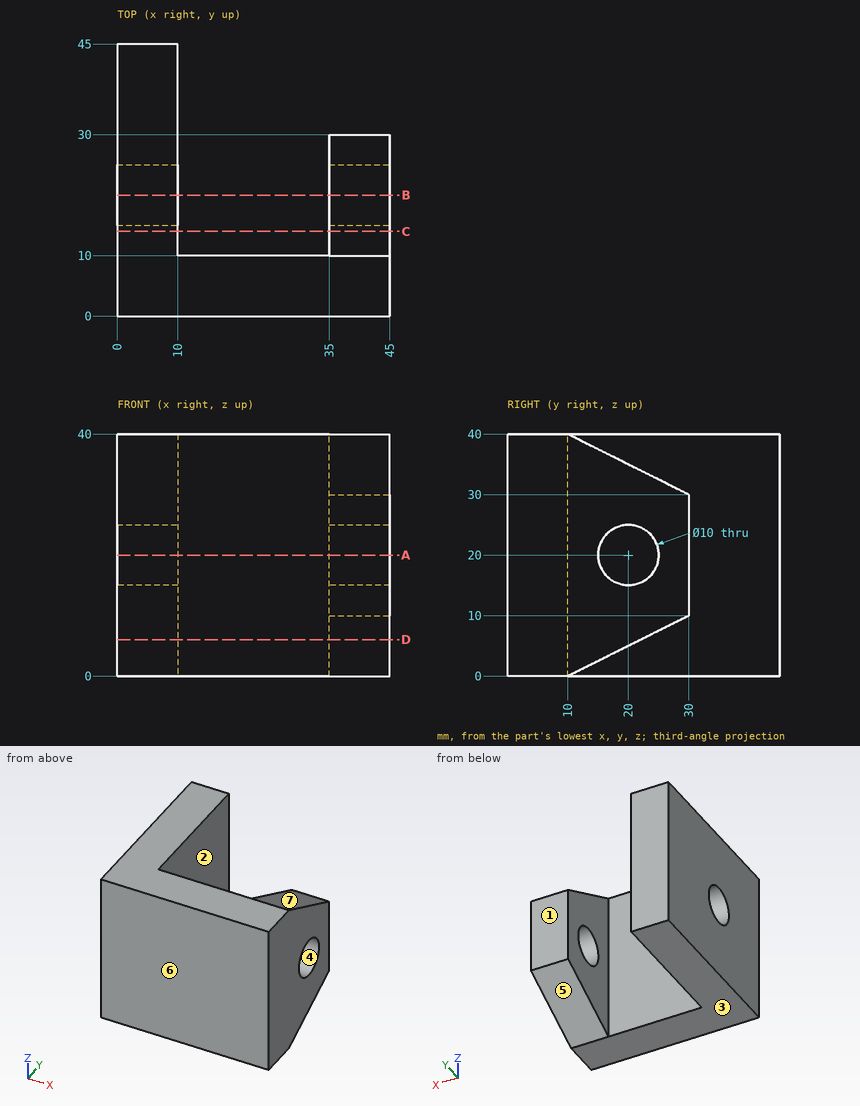
The drawing under review shows one solid part. Ordinate dimensions are in mm from its lowest x, y, z. A direction names the side the tool comes from. Round coordinates to 2 decimals unless told otherwise and drop trailing zeros. Order: outer loops, then holes, each group sorted by start corner. A loop starts at its lowest first (then second) coordinate and runs counter-clockwise, first axis right, second up. Notation, with made-up numbers: (5.5, -36) -> (64.5, -36) arc R34 ccw to (64.5, -4) -> close; hole circle Ø6 at (59, 63). An arc over 180 degrees is marked (long way). Use a Markdown table: item, result.
Q1. Tool access review of the marked faces 1, 2 and 3: name each direction out of +Z, -Z, +X, -X, +Y, -Y from which nothing blocks a thin tool from reaching the whole face with its end or side.
Values:
| item | result |
|---|---|
| face 1 | +Z, -Z, +X, +Y |
| face 2 | +Z, -Z, +Y |
| face 3 | -Z, +X, -X, +Y, -Y |
Q2. For line 1 (X direction, y = 12.5, z = 9.5); line 2 (Z direction, x = 4, y = 20); line 3 (Y direction, x = 4, z = 20), list the stretches that pass through material, from the lowest coordinate up.
Values:
| item | result |
|---|---|
| line 1 | x = 0 to 10, 35 to 45 |
| line 2 | z = 0 to 15, 25 to 40 |
| line 3 | y = 0 to 15, 25 to 45 |
Q3. We need section B-B on y = 20. Write out the cut boundary in (x, z).
Values:
| item | result |
|---|---|
| outline | (0, 0) -> (10, 0) -> (10, 15) -> (0, 15) -> close; (0, 25) -> (10, 25) -> (10, 40) -> (0, 40) -> close; (35, 5) -> (45, 5) -> (45, 15) -> (35, 15) -> close; (35, 25) -> (45, 25) -> (45, 35) -> (35, 35) -> close |
Q4. Clearance check with flat-ended pins moving along their axes: P1, Ø10, axis at x = 28, z = 31, coming from the +Y side; P2, Ø8, axis at y = 20, z = 20, coming from the +X side; P3, Ø4, axis at x = 37, y = 31.5, coming from the -Z side; P4, Ø5, axis at x = 39, z = 15, coming from the +Y side. State where each tip first meets the part, or that it passes through.
Values:
| item | result |
|---|---|
| P1 | stops at y = 10 |
| P2 | passes through |
| P3 | stops at z = 9.75 |
| P4 | stops at y = 30 |
Q5. We need section C-C on y = 14. Write out the cut boundary in (x, z).
Values:
| item | result |
|---|---|
| outline | (0, 0) -> (10, 0) -> (10, 40) -> (0, 40) -> close; (35, 2) -> (45, 2) -> (45, 38) -> (35, 38) -> close |
Q6. We need section A-A on z = 20. Write out the cut boundary in (x, y), then the cut area to 3 significant figures.
Values:
| item | result |
|---|---|
| outline | (0, 0) -> (45, 0) -> (45, 15) -> (35, 15) -> (35, 10) -> (10, 10) -> (10, 15) -> (0, 15) -> close; (0, 25) -> (10, 25) -> (10, 45) -> (0, 45) -> close; (35, 25) -> (45, 25) -> (45, 30) -> (35, 30) -> close |
| area | 800 mm^2 |
Q7. We need section D-D on z = 6. Write out the cut boundary in (x, y), then the cut area to 3 significant figures.
Values:
| item | result |
|---|---|
| outline | (0, 0) -> (45, 0) -> (45, 22) -> (35, 22) -> (35, 10) -> (10, 10) -> (10, 45) -> (0, 45) -> close |
| area | 920 mm^2 |
Q8. Mouldability with a two-part tool opening along Z and no side actions: class the marked faces 4, 5, 6 and 7 as +Z half, -Z half, draft (parallel to the pull), parting line (faces both ways), or undercut.
Values:
| item | result |
|---|---|
| face 4 | undercut |
| face 5 | -Z half |
| face 6 | draft |
| face 7 | +Z half |
